```python
from build123d import *

# Parameters (mm, degrees)
BOSS_EXTRUDE1_DEPTH      = 2.5
BOSS_EXTRUDE2_DEPTH      = 8.5
BOSS_EXTRUDE2_DEPTH_BACK = 3.25
SKETCH2_W                = 0.75
SKETCH2_H                = 0.75
CHAMFER1_SIZE            = 0.3


with BuildPart() as part:
    # Sketch1 → Boss-Extrude1 (new body)
    with BuildSketch(Plane(origin=(0, 0, 0), x_dir=(-1, 0, 0), z_dir=(0, 1, 0))):
        with BuildLine():
            Line((-3.27, 1.27), (3.27, 1.27))
            ThreePointArc((3.27, 1.27), (3.623553391, 1.123553391), (3.77, 0.77))
            Line((3.77, 0.77), (3.77, -0.77))
            ThreePointArc((3.77, -0.77), (3.623553391, -1.123553391), (3.27, -1.27))
            Line((3.27, -1.27), (-3.27, -1.27))
            ThreePointArc((-3.27, -1.27), (-3.623553391, -1.123553391), (-3.77, -0.77))
            Line((-3.77, -0.77), (-3.77, 0.77))
            ThreePointArc((-3.77, 0.77), (-3.623553391, 1.123553391), (-3.27, 1.27))
        make_face()
    extrude(amount=BOSS_EXTRUDE1_DEPTH)

    # Sketch2 → Boss-Extrude2 (add, two sides: drawn at the far end of the back side and taken through both)
    with BuildSketch(Plane(origin=(0, 0, 0), x_dir=(-1, 0, 0), z_dir=(0, 1, 0)).offset(-BOSS_EXTRUDE2_DEPTH_BACK)):
        with Locations((2.54, 0)):
            Rectangle(SKETCH2_W, SKETCH2_H)
        Rectangle(SKETCH2_W, SKETCH2_H)
        with Locations((-2.54, 0)):
            Rectangle(SKETCH2_W, SKETCH2_H)
    extrude(amount=BOSS_EXTRUDE2_DEPTH + BOSS_EXTRUDE2_DEPTH_BACK)

    # Chamfer1
    chamfer1_edges = [part.edges().sort_by_distance(p)[0] for p in [
        (-2.165, -3.25, 0),
        (-2.54, -3.25, 0.375),
        (-2.915, -3.25, 0),
        (-2.54, -3.25, -0.375),
        (-2.165, 8.5, 0),
        (-2.54, 8.5, -0.375),
        (-2.915, 8.5, 0),
        (-2.54, 8.5, 0.375),
        (-0.375, -3.25, 0),
        (0, -3.25, -0.375),
        (0.375, -3.25, 0),
        (0, -3.25, 0.375),
        (-0.375, 8.5, 0),
        (0, 8.5, 0.375),
        (0.375, 8.5, 0),
        (0, 8.5, -0.375),
        (2.165, -3.25, 0),
        (2.54, -3.25, -0.375),
        (2.915, -3.25, 0),
        (2.54, -3.25, 0.375),
        (2.165, 8.5, 0),
        (2.54, 8.5, 0.375),
        (2.915, 8.5, 0),
        (2.54, 8.5, -0.375),
    ]]
    chamfer(chamfer1_edges, length=CHAMFER1_SIZE)


solid = part.part
```
The model under review builds one solid part; all positions refer to its coordinate system, in mm. Round coordinates to 2 decimals unless told otherwise and drop trailing zeros. Order: outer loops, then holes, each group sorted by start corner. A loop starts at its lowest first (then second) coordinate and runs counter-clockwise, first axis right, second up.
Item 1: Add section C-C, the plane z = 0.55. State the section outline as (x, y) points.
Working result:
outline: (-3.77, 0) - (3.77, 0) - (3.77, 2.5) - (-3.77, 2.5) - close
Item 2: Add section B-B, the plane x = -2. State the section outline as (y, z) points, and give its area (3 significant figures).
Working result:
outline: (0, -1.27) - (2.5, -1.27) - (2.5, 1.27) - (0, 1.27) - close
area: 6.35 mm2
Item 3: Add section D-D, the plane x = 0.25. State the section outline as (y, z) points (3 decimals).
Working result:
outline: (-3.075, -0.25) - (-2.95, -0.375) - (0, -0.375) - (0, -1.27) - (2.5, -1.27) - (2.5, -0.375) - (8.2, -0.375) - (8.325, -0.25) - (8.325, 0.25) - (8.2, 0.375) - (2.5, 0.375) - (2.5, 1.27) - (0, 1.27) - (0, 0.375) - (-2.95, 0.375) - (-3.075, 0.25) - close
Item 4: For pin 1 (0.6 mm diameter, centred on y = 5, z = 0, fed in from -X) (3 decimals); pin 2 (1.5 mm diameter, centred on x = 2, y = 5.5, fed in from -Z) (3 decimals); pin 3 (0.8 mm diameter, centred on y = 5.5, z = 0, fed in from +X) (3 decimals), all flat-tipped, find the tip position at first contact; note any pin that passes through.
Working result:
pin 1: stops at x = -2.915
pin 2: stops at z = -0.375
pin 3: stops at x = 2.915
Item 5: To check wall thickness, follow probe 1 along X at (y, z) = (5.75, 0.3) (3 decimals); probe 2 along Y at (x, z) = (0.5, 0.95); probe 3 along Z at (x, y) = (2.75, 3.75) (3 decimals). State the ranges of each line that lie inside material, in increasing order.
Working result:
probe 1: x = -2.915 to -2.165, -0.375 to 0.375, 2.165 to 2.915
probe 2: y = 0 to 2.5
probe 3: z = -0.375 to 0.375
Item 6: Add section A-A, the plane y = 6.5. State the section outline as (x, z) points (3 decimals), and give its area (3 significant figures).
Working result:
outline: (-2.915, -0.375) - (-2.165, -0.375) - (-2.165, 0.375) - (-2.915, 0.375) - close; (-0.375, -0.375) - (0.375, -0.375) - (0.375, 0.375) - (-0.375, 0.375) - close; (2.165, -0.375) - (2.915, -0.375) - (2.915, 0.375) - (2.165, 0.375) - close
area: 1.69 mm2
